```python
from build123d import *

# Parameters (mm, degrees)
SKETCH1_R           = 63.5
SKETCH1_R_2         = 2.286
BOSS_EXTRUDE1_DEPTH = 50.8
SKETCH2_R           = 12.7
CUT_EXTRUDE1_DEPTH  = 51.8


with BuildPart() as part:
    # Sketch1 → Boss-Extrude1 (new body)
    with BuildSketch(Plane.XY):
        Circle(SKETCH1_R)
        with Locations((-33.02, 0)):
            Circle(SKETCH1_R_2, mode=Mode.SUBTRACT)
        with Locations((33.02, 0)):
            Circle(SKETCH1_R_2, mode=Mode.SUBTRACT)
        with Locations((0, 38.862)):
            Circle(SKETCH1_R_2, mode=Mode.SUBTRACT)
    extrude(amount=BOSS_EXTRUDE1_DEPTH)

    # Sketch2 → Cut-Extrude1 (cut, through all)
    with BuildSketch(Plane.XY.offset(50.8)):
        Circle(SKETCH2_R)
    extrude(amount=-CUT_EXTRUDE1_DEPTH, mode=Mode.SUBTRACT)


solid = part.part
```
Work out the finished part from the listing and answer in its coordinate system (mm). Coordinates: 2 decimals unless noted, no trailing zeros. Write each loop counter-clockwise with the first axis right and the second up, starting at its lowest first coordinate (ties: lowest second). Pieces come first, ordered by that corner, then holes.
Q1. A cutting plane is placed at D-D, the plane x = -17.5. Give the vertices of the cut face in (y, z), then the cut area to 3 significant figures.
Q2. Each of these flat-tipped pins is pushed along its axis until it touches: pin 1 Ø8 at (y, z) = (-28.5, 9) entering from -X; pin 2 Ø5 at (y, z) = (38.5, 34.5) entering from -X; pin 3 Ø4 at (y, z) = (-9.5, 34.5) entering from +X. Where does it stop, or does it pass through?
Q3. Determine the mould class of faces 1 (the face through (13, 1, 50.8)), 2 (the face through (-30.91, -0.88, 25.04)), 3 (the face through (-13.77, -61.99, 25.04)) for opening direction Y: released by +Y, released by -Y, zero draft, split by the parting line, or undercut.
Q4. A cutting plane is placed at A-A, the plane x = 0. Give the vertices of the cut face in (y, z), then the cut area to 3 significant figures.
Q5. A cutting plane is placed at B-B, the plane y = 0. Give the vertices of the cut face in (x, z), then the cut area to 3 significant figures.
Q6. Find the intervals of material crossed by line 1 (X direction, y = 2, z = 16.5); line 2 (X direction, y = 7, z = 36); line 3 (X direction, y = 9.5, z = 8), in increasing order.
Q7. A cutting plane is placed at C-C, the plane x = -33.02. Give the vertices of the cut face in (y, z), then the cut area to 3 significant figures.
Findings below:
1. outline: (-61.04, 0) - (61.04, 0) - (61.04, 50.8) - (-61.04, 50.8) - close
1. area: 6,200 mm2
2. pin 1: stops at x = -58.58
2. pin 2: stops at x = -52.31
2. pin 3: stops at x = 63.06
3. face 1: zero draft
3. face 2: undercut
3. face 3: split by the parting line
4. outline: (-63.5, 0) - (-12.7, 0) - (-12.7, 50.8) - (-63.5, 50.8) - close; (12.7, 0) - (36.58, 0) - (36.58, 50.8) - (12.7, 50.8) - close; (41.15, 0) - (63.5, 0) - (63.5, 50.8) - (41.15, 50.8) - close
4. area: 4,930 mm2
5. outline: (-63.5, 0) - (-35.31, 0) - (-35.31, 50.8) - (-63.5, 50.8) - close; (-30.73, 0) - (-12.7, 0) - (-12.7, 50.8) - (-30.73, 50.8) - close; (12.7, 0) - (30.73, 0) - (30.73, 50.8) - (12.7, 50.8) - close; (35.31, 0) - (63.5, 0) - (63.5, 50.8) - (35.31, 50.8) - close
5. area: 4,700 mm2
6. line 1: x = -63.47 to -34.13, -31.91 to -12.54, 12.54 to 31.91, 34.13 to 63.47
6. line 2: x = -63.11 to -10.6, 10.6 to 63.11
6. line 3: x = -62.79 to -8.43, 8.43 to 62.79
7. outline: (-54.24, 0) - (-2.29, 0) - (-2.29, 50.8) - (-54.24, 50.8) - close; (2.29, 0) - (54.24, 0) - (54.24, 50.8) - (2.29, 50.8) - close
7. area: 5,280 mm2
